Read the model definition and answer for the solid it produces. Units are mm, in the model's axes. A direction names the side the tool comes from. Coordinates: 2 decimals unless noted, no trailing zeros. Loops run counter-clockwise (first coordinate to the right, second up) from the corner with the lowest first, then second, coordinate; pieces in that order, holes last.
from build123d import *

# Parameters (mm, degrees)
F1_DEPTH = 3.175
F3_D     = 19.05


with BuildPart() as f1:
    # F0 (on Front) → F1 (new body, symmetric)
    with BuildSketch(Plane.XZ):
        Polygon((25.4, 177.8), (0, 177.8), (0, -25.4), (127, -25.4), (127, 0), (50.8, 0), align=None)
    extrude(amount=F1_DEPTH, both=True)

    # F3 (through all)
    with Locations(Plane.XZ.offset(3.175)):
        with Locations((18.947579, 75.414784), (19.903496, 20.927686)):
            Hole(F3_D / 2)


solid = f1.part
Q1. Determine the mould class of faces 1 (the face through (27.46, 0.04, 15.13)), 2 (the face through (34, -3.175, 55)), 3 (the face through (21.012, 0.044, 66.116)), 4 (the face through (127, 0, -13)) for opening direction X: +X half, -X half, draft (parallel to the pull), parting line (faces both ways), or undercut.
Findings below:
face 1: undercut
face 2: draft
face 3: undercut
face 4: +X half
Q2. A cutting plane is placed at A-A (x = 15). Give the vertices of the cut face in (y, z) (3 decimals), then the cut area to 3 significant figures.
Findings below:
outline: (-3.175, -25.4) - (3.175, -25.4) - (3.175, 12.762) - (-3.175, 12.762) - close; (-3.175, 29.094) - (3.175, 29.094) - (3.175, 66.746) - (-3.175, 66.746) - close; (-3.175, 84.083) - (3.175, 84.083) - (3.175, 177.8) - (-3.175, 177.8) - close
area: 1,080 mm2
Q3. A cutting plane is placed at D-D (z = 111). Give the vertices of the cut face in (x, y) (3 decimals), then the cut area to 3 significant figures.
Findings below:
outline: (0, -3.175) - (34.943, -3.175) - (34.943, 3.175) - (0, 3.175) - close
area: 222 mm2
Q4. A cutting plane is placed at B-B (y = -0.75). Count the separate pieces of the cut face and the enclosed holes in it, then the cut area to 3 significant figures.
Findings below:
separate pieces: 1
enclosed holes: 2
area: 9,430 mm2
Q5. Straight lines are drawn through the part: probe 1 along Z at (x, y) = (73, -2.5); probe 2 along Z at (x, y) = (14, 0.75); probe 3 along X at (y, z) = (-1.5, 70.5). For each, find the intervals that lie inside material, in ascending order.
Findings below:
probe 1: z = -25.4 to 0
probe 2: z = -25.4 to 13.45, 28.4 to 67.28, 83.55 to 177.8
probe 3: x = 0 to 10.79, 27.11 to 40.73
Q6. Flat-ended cylindrical pins translate along their axes: pin 1 Ø3 at (y, z) = (-2.5, 15) entering from +X; pin 2 Ø17 at (x, z) = (19.9, 20.93) entering from +Y. Find the tip coordinate at first contact, or state that the pin passes through.
Findings below:
pin 1: stops at x = 48.87
pin 2: passes through
Q7. A cutting plane is placed at C-C (x = 54.5). Give the vertices of the cut face in (y, z) (3 decimals), then the cut area to 3 significant figures.
Findings below:
outline: (-3.175, -25.4) - (3.175, -25.4) - (3.175, 0) - (-3.175, 0) - close
area: 161 mm2
Q8. Which of the six approach directions +Z, -Z, +X, -X, +Y, -Y give full straight-line access (tool end or side, diameter ignored) to faces 5 (the face through (0, 0, 78)), 6 (the face through (89, 0, 0))?
Findings below:
face 5: +Z, -Z, -X, +Y, -Y
face 6: +Z, +X, +Y, -Y
